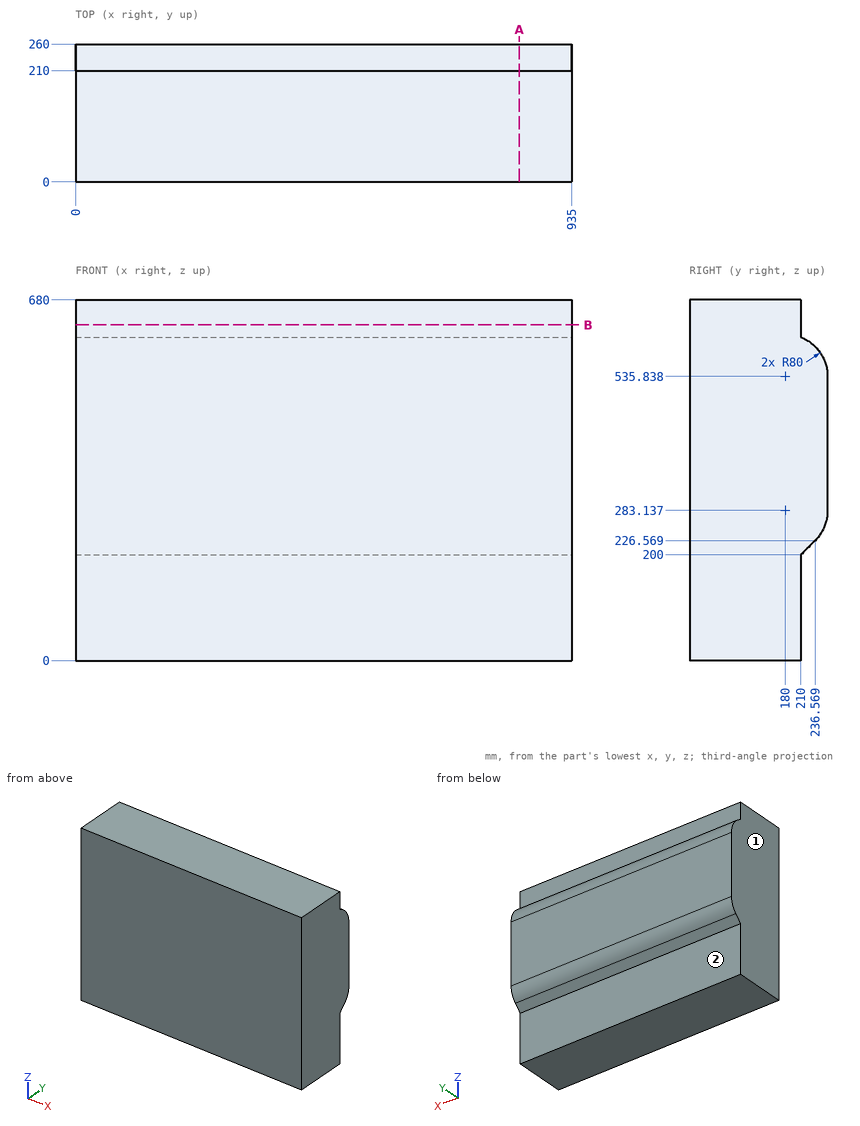
Verification items for this drawing (mm, ordinates from the low corner). A direction names the side the tool comes from. Coordinates: 2 decimals unless noted, no trailing zeros. Loops run counter-clockwise (first coordinate to the right, second up) from the corner with the lowest first, then second, coordinate; pieces in that order, holes last.
Item 1: Sectioned sample at B-B, the plane z = 633. Record the boundary of the cut face in (x, y), then the cut area to 3 significant figures.
Item 2: Thickness scan on line 1 (Y direction, x = 671.5, z = 118.5); line 2 (Z direction, x = 642.5, y = 236.5) (1 decimal); line 3 (Y direction, x = 792, z = 600.5) (1 decimal). Record the ranges inside material, lowest first.
Item 3: Sectioned sample at A-A, the plane x = 836.5. Record the boundary of the cut face in (y, z).
Item 4: Access from +Z, -Z, +X, -X, +Y, -Y to the whole of each face (thin tool, end or side, straight path). Record for the marked faces 1 and 2.
Item 5: Go/stop test with a flat-tipped pin: pin 1 Ø1.5 at (x, y) = (738, 233) entering from +Z. Record where the tip stops, or that it passes through.
Check result:
1. outline: (0, 0) - (935, 0) - (935, 210) - (0, 210) - close
1. area: 196,000 mm2
2. line 1: y = 0 to 210
2. line 2: z = 226.5 to 592.5
2. line 3: y = 0 to 227.1
3. outline: (0, 0) - (210, 0) - (210, 200) - (236.57, 226.57) arc R80 ccw to (260, 283.14) - (260, 535.84) arc R80 ccw to (210, 610) - (210, 680) - (0, 680) - close
4. face 1: +Z, -Z, -X, +Y, -Y
4. face 2: -Z, +X, -X, +Y
5. pin 1: stops at z = 596.42
